```python
from build123d import *

# Parameters (mm, degrees)
EXTRUDE_1_DEPTH          = 27
EXTRUDE_1_DEPTH_BACK     = 4
SKETCH_1_W               = 53
SKETCH_1_H               = 30.25
SKETCH_2_W               = 49
SKETCH_2_H               = 26.25
CUT_EXTRUDE_1_DEPTH      = 28.2
SKETCH_3_W               = 52
SKETCH_3_H               = 29.25
SKETCH_3_W_2             = 50.4
SKETCH_3_H_2             = 27.65
CUT_EXTRUDE_2_DEPTH      = 1
CUT_EXTRUDE_3_REACH      = 45.497
SKETCH_4_R               = 1
SKETCH_5_R               = 1.55
CUT_EXTRUDE_4_DEPTH      = 1
MIRROR_2_COPY_1_REACH    = 45.497
MIRROR_2_COPY_1_SKETCH_R = 1
MIRROR_2_COPY_2_SKETCH_R = 1.55
MIRROR_2_COPY_2_DEPTH    = 1
SKETCH_7_R               = 2
CUT_EXTRUDE_6_DEPTH      = 60.655390578
SKETCH_8_W               = 52
SKETCH_8_H               = 29.25
SKETCH_8_W_2             = 50.4
SKETCH_8_H_2             = 27.65
EXTRUDE_2_DEPTH          = 1.5


with BuildPart() as part:
    # 草图1 → 凸台-拉伸1 (new, two sides: drawn at the far end of the back side and taken through both)
    with BuildSketch(Plane.XY.offset(-EXTRUDE_1_DEPTH_BACK)):
        Rectangle(SKETCH_1_W, SKETCH_1_H)
    extrude(amount=EXTRUDE_1_DEPTH + EXTRUDE_1_DEPTH_BACK)

    # 草图2 → 切除-拉伸1 (cut)
    with BuildSketch(Plane.XY.offset(27)):
        Rectangle(SKETCH_2_W, SKETCH_2_H)
    extrude(amount=-CUT_EXTRUDE_1_DEPTH, mode=Mode.SUBTRACT)

    # 草图3 → 切除-拉伸2 (cut)
    with BuildSketch(Plane.XY.offset(27)):
        Rectangle(SKETCH_3_W, SKETCH_3_H)
        Rectangle(SKETCH_3_W_2, SKETCH_3_H_2, mode=Mode.SUBTRACT)
    extrude(amount=-CUT_EXTRUDE_2_DEPTH, mode=Mode.SUBTRACT)

    # 草图4 → 切除-拉伸3 (cut, up to next)
    with BuildSketch(Plane(origin=(0, 0, -4), x_dir=(-1, 0, 0), z_dir=(0, 0, -1)), mode=Mode.PRIVATE) as cut_extrude_3_sk1:
        with Locations((-22.65, 11.275)):
            Circle(SKETCH_4_R)
    cut_extrude_3_tool1 = extrude(cut_extrude_3_sk1.sketch, amount=-CUT_EXTRUDE_3_REACH, mode=Mode.PRIVATE) & part.part
    cut_extrude_3 = cut_extrude_3_tool1.solids().sort_by_distance((22.65, 11.275, -4))[0]
    add(cut_extrude_3, mode=Mode.SUBTRACT)

    # 草图5 → 切除-拉伸4 (cut)
    with BuildSketch(Plane(origin=(0, 0, -4), x_dir=(-1, 0, 0), z_dir=(0, 0, -1))):
        with Locations((-22.65, 11.275)):
            Circle(SKETCH_5_R)
    cut_extrude_4 = extrude(amount=-CUT_EXTRUDE_4_DEPTH, mode=Mode.SUBTRACT)

    # 镜向1: 切除-拉伸3, 切除-拉伸4 across plane
    add(cut_extrude_3.mirror(Plane.ZX), mode=Mode.SUBTRACT)
    add(cut_extrude_4.mirror(Plane.ZX), mode=Mode.SUBTRACT)

    # 镜向2: 切除-拉伸3, 切除-拉伸4 across plane
    add(cut_extrude_3.mirror(Plane(origin=(0, 0, 0), x_dir=(0, 0, 1), z_dir=(1, 0, 0))), mode=Mode.SUBTRACT)
    add(cut_extrude_4.mirror(Plane(origin=(0, 0, 0), x_dir=(0, 0, 1), z_dir=(1, 0, 0))), mode=Mode.SUBTRACT)

    # 镜向2 copy 1 sketch → 镜向2 copy 1 (cut, up to next)
    with BuildSketch(Plane(origin=(0, 0, -4), x_dir=(1, 0, 0), z_dir=(0, 0, -1)), mode=Mode.PRIVATE) as mirror_2_copy_1_sk1:
        with Locations((-22.65, 11.275)):
            Circle(MIRROR_2_COPY_1_SKETCH_R)
    mirror_2_copy_1_tool1 = extrude(mirror_2_copy_1_sk1.sketch, amount=-MIRROR_2_COPY_1_REACH, mode=Mode.PRIVATE) & part.part
    add(mirror_2_copy_1_tool1.solids().sort_by_distance((-22.65, -11.275, -4))[0], mode=Mode.SUBTRACT)

    # 镜向2 copy 2 sketch → 镜向2 copy 2 (cut)
    with BuildSketch(Plane(origin=(0, 0, -4), x_dir=(1, 0, 0), z_dir=(0, 0, -1))):
        with Locations((-22.65, 11.275)):
            Circle(MIRROR_2_COPY_2_SKETCH_R)
    extrude(amount=-MIRROR_2_COPY_2_DEPTH, mode=Mode.SUBTRACT)

    # 草图7 → 切除-拉伸6 (cut, through all)
    with BuildSketch(Plane.ZY.offset(-24.5)):
        with Locations((8.54820427, 0)):
            Circle(SKETCH_7_R)
    extrude(amount=-CUT_EXTRUDE_6_DEPTH, mode=Mode.SUBTRACT)

    # 草图8 → 凸台-拉伸2 (add)
    with BuildSketch(Plane.XY.offset(26)):
        Rectangle(SKETCH_8_W, SKETCH_8_H)
        Rectangle(SKETCH_8_W_2, SKETCH_8_H_2, mode=Mode.SUBTRACT)
    extrude(amount=EXTRUDE_2_DEPTH)


solid = part.part
```
Could you check a few things on this model? Use its own coordinates, in mm. A direction names the side the tool comes from. Give positions to 0.01 mm unless a question says otherwise; leave off trailing zeros. Loops run counter-clockwise (first coordinate to the right, second up) from the corner with the lowest first, then second, coordinate; pieces in that order, holes last. Notation, with made-up numbers: (-32, 80) -> (19, 80) arc R23 ccw to (19, 116) -> close; hole circle Ø5 at (61.25, 45). An arc over 180 degrees is marked (long way). Put each result on its own line as item: value.
(1) Thinking about a two-plate mould opening in Y: for faces 1 (the face through (0, -15.125, 11)), 2 (the face through (0, 0, -4)), 3 (the face through (25.49, 0.09, 6.55)), which applies, pulls with the +Y half, pulls with the -Y half, needs draft (parallel to the pull), parting line crosses it, or undercut?
Computed:
face 1: pulls with the -Y half
face 2: needs draft
face 3: undercut
(2) Imagine slicing it at C-C on y = 0. Write out the boundary of the cut face in (x, z), plus the area to 3 significant figures.
Computed:
outline: (-26.5, -4) -> (26.5, -4) -> (26.5, 6.55) -> (24.5, 6.55) -> (24.5, -1.2) -> (-24.5, -1.2) -> (-24.5, 27) -> (-25.2, 27) -> (-25.2, 27.5) -> (-26, 27.5) -> (-26, 27) -> (-26.5, 27) -> close; (24.5, 10.55) -> (26.5, 10.55) -> (26.5, 27) -> (26, 27) -> (26, 27.5) -> (25.2, 27.5) -> (25.2, 27) -> (24.5, 27) -> close
area: 254 mm^2
(3) Please list where these lines run through material, in increasing order: probe 1 along Y at (x, z) = (22.65, -2.4) (3 decimals); probe 2 along Y at (x, z) = (22.65, -3.4) (3 decimals); probe 3 along Y at (x, z) = (-20.5, 4) (3 decimals). Write a range as [from, to].
Computed:
probe 1: [-15.125, -12.275], [-10.275, 10.275], [12.275, 15.125]
probe 2: [-15.125, -12.825], [-9.725, 9.725], [12.825, 15.125]
probe 3: [-15.125, -13.125], [13.125, 15.125]
(4) Imagine slicing it at D-D on x = -12. Write out the boundary of the cut face in (y, z) (3 decimals).
Computed:
outline: (-15.125, -4) -> (15.125, -4) -> (15.125, 27) -> (14.625, 27) -> (14.625, 27.5) -> (13.825, 27.5) -> (13.825, 27) -> (13.125, 27) -> (13.125, -1.2) -> (-13.125, -1.2) -> (-13.125, 27) -> (-13.825, 27) -> (-13.825, 27.5) -> (-14.625, 27.5) -> (-14.625, 27) -> (-15.125, 27) -> close
(5) Imagine slicing it at B-B on z = 21.5. Write out the boundary of the cut face in (x, y) (3 decimals).
Computed:
outline: (-26.5, -15.125) -> (26.5, -15.125) -> (26.5, 15.125) -> (-26.5, 15.125) -> close; hole (-24.5, -13.125) -> (24.5, -13.125) -> (24.5, 13.125) -> (-24.5, 13.125) -> close
(6) I'm going to push flat-ended pins straight in: pin 1 Ø5 at (x, y) = (-7.5, -9.5) entering from +Z; pin 2 Ø0.6 at (y, z) = (5.5, 27.5) entering from +X; pin 3 Ø2.5 at (x, y) = (-22.65, -11.275) entering from -Z; pin 4 Ø1.9 at (x, y) = (-22.65, 11.275) entering from -Z. Where does each tip first touch, or does it pass through?
Computed:
pin 1: z = -1.2
pin 2: x = 26
pin 3: z = -3
pin 4: through
(7) Imagine slicing it at A-A on x = -22.65. State how many separate pieces and enclosed holes the cut face has, plus the area to 3 significant figures.
Computed:
separate pieces: 3
enclosed holes: 0
area: 185 mm^2
(8) For faces 4 (the face through (-23.39, 11.95, -2.11)), 5 (the face through (21.22, -10.68, -3.51)), 6 (the face through (0, 13.125, 13)), which set-ups out of +Z, -Z, +X, -X, +Y, -Y let a thin tool reach every point of the face, with its end or its side?
Computed:
face 4: +Z, -Z
face 5: -Z
face 6: +Z
